Source: three-view drawing plus pictorial views. Frame: mm from the lowest corner of the part. A direction names the side the tool comes from. Give positions to 0.01 mm unless a question says otherwise; leave off trailing zeros. Loops run counter-clockwise (first coordinate to the right, second up) from the corner with the lowest first, then second, coordinate; pieces in that order, holes last. Notation, with made-up numbers: (81.25, 4) -> (124.25, 4) arc R11 ccw to (124.25, 18) -> close; hole circle Ø10 at (29.5, 30). An arc over 180 degrees is marked (long way). Put each result on its own line as item: value.
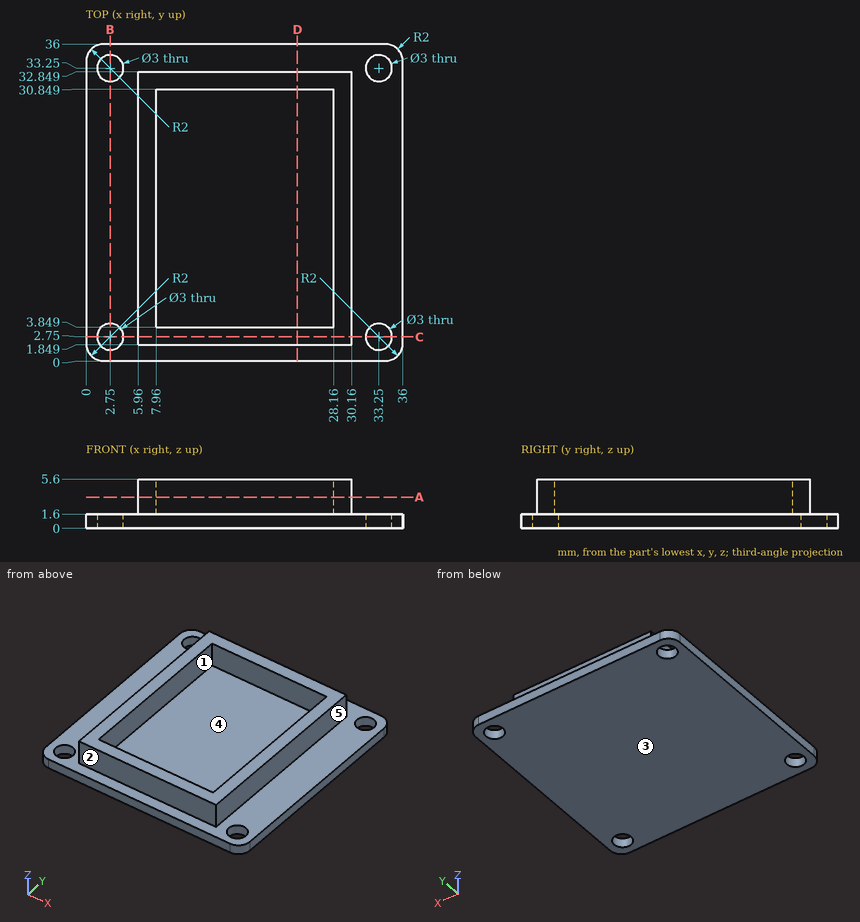
(1) Section D-D on x = 24. Return loops of the section in (y, z).
Calculated:
outline: (0, 0) -> (36, 0) -> (36, 1.6) -> (32.85, 1.6) -> (32.85, 5.6) -> (30.85, 5.6) -> (30.85, 1.6) -> (3.85, 1.6) -> (3.85, 5.6) -> (1.85, 5.6) -> (1.85, 1.6) -> (0, 1.6) -> close
(2) Reachability of the marked faces 4 and 5 from +Z, -Z, +X, -X, +Y, -Y: full face, straight path, thin tool, end or side. Return the list, or none.
Calculated:
face 4: +Z
face 5: +Z, +X, +Y, -Y
(3) First-contact query: P1, Ø1.2, axis at x = 16.5, z = 2.5, coming from the -Y side; P2, Ø10, axis at x = 17.5, y = 13.5, coming from the +Z side; P3, Ø2, axis at y = 13.5, z = 2.5, coming from the +X side; P4, Ø1, axis at y = 17.5, z = 2.5, coming from the +X side. Flat tips, straight axial feed; report the tip coordinate or a pass-through.
Calculated:
P1: stops at y = 1.85
P2: stops at z = 1.6
P3: stops at x = 36
P4: stops at x = 30.16
(4) Section A-A on z = 3.55. Return loops of the section in (x, y).
Calculated:
outline: (5.96, 1.85) -> (30.16, 1.85) -> (30.16, 32.85) -> (5.96, 32.85) -> close; hole (7.96, 3.85) -> (28.16, 3.85) -> (28.16, 30.85) -> (7.96, 30.85) -> close
(5) Section C-C on y = 2.75. Return loops of the section in (x, z).
Calculated:
outline: (0, 0) -> (1.25, 0) -> (1.25, 1.6) -> (0, 1.6) -> close; (4.25, 0) -> (31.75, 0) -> (31.75, 1.6) -> (30.16, 1.6) -> (30.16, 5.6) -> (5.96, 5.6) -> (5.96, 1.6) -> (4.25, 1.6) -> close; (34.75, 0) -> (36, 0) -> (36, 1.6) -> (34.75, 1.6) -> close
(6) Section B-B on x = 2.75. Return loops of the section in (y, z).
Calculated:
outline: (0, 0) -> (1.25, 0) -> (1.25, 1.6) -> (0, 1.6) -> close; (4.25, 0) -> (31.75, 0) -> (31.75, 1.6) -> (4.25, 1.6) -> close; (34.75, 0) -> (36, 0) -> (36, 1.6) -> (34.75, 1.6) -> close
(7) Line query: probe 1 along Y at (x, z) = (2.75, 0.4); probe 2 along X at (y, z) = (11, 4.2); probe 3 along Y at (x, z) = (11, 4.65). Output: solid intervals per line, ascending. Write a range as from..to.
Calculated:
probe 1: y = 0..1.25, 4.25..31.75, 34.75..36
probe 2: x = 5.96..7.96, 28.16..30.16
probe 3: y = 1.85..3.85, 30.85..32.85
(8) Draft query along Y for the marked faces 1, 2 and 3. Return one class per face: released by +Y, released by -Y, zero draft, split by the parting line, or undercut.
Calculated:
face 1: undercut
face 2: released by -Y
face 3: zero draft
